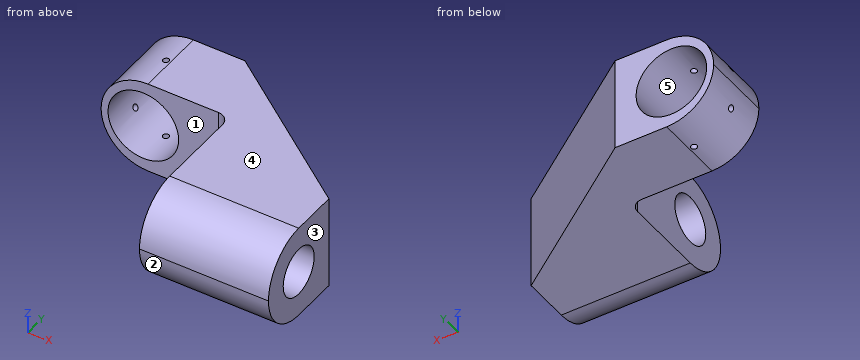
```python
from build123d import *

# Parameters (mm, degrees)
BOSS_EXTRUDE1_DEPTH     = 40
FILLET1_R               = 5
CUT_EXTRUDE1_REACH      = 114.805
SKETCH2_R               = 10.25
CUT_EXTRUDE2_REACH      = 133.529
SKETCH3_R               = 15.05
FILLET3_R               = 20
CUT_EXTRUDE5_DEPTH      = 37
CUT_EXTRUDE5_DEPTH_BACK = 7
SKETCH7_R               = 1.325
CUT_EXTRUDE7_DEPTH      = 7
CUT_EXTRUDE7_DEPTH_BACK = 7
SKETCH8_R               = 1.325
CUT_EXTRUDE8_DEPTH      = 7
CUT_EXTRUDE8_DEPTH_BACK = 7
SKETCH9_R               = 1.325
FILLET4_START           = -30
FILLET4_DEPTH           = 30


with BuildPart() as part:
    # Sketch1 → Boss-Extrude1 (new body)
    with BuildSketch(Plane.XY):
        Polygon((0, 0), (42, 0), (110, -50), (110, -90), (55, -90), (55, -30), (0, -30), align=None)
    extrude(amount=BOSS_EXTRUDE1_DEPTH)

    # Fillet1
    fillet1_edges = [part.edges().sort_by_distance(p)[0] for p in [
        (55, -30, 20),
    ]]
    fillet(fillet1_edges, radius=FILLET1_R)

    # Sketch2 → Cut-Extrude1 (cut, up to next)
    with BuildSketch(Plane.ZY.offset(-55), mode=Mode.PRIVATE) as cut_extrude1_sk1:
        with Locations((20, -70)):
            Circle(SKETCH2_R)
    cut_extrude1_tool1 = extrude(cut_extrude1_sk1.sketch, amount=-CUT_EXTRUDE1_REACH, mode=Mode.PRIVATE) & part.part
    add(cut_extrude1_tool1.solids().sort_by_distance((55, -70, 20))[0], mode=Mode.SUBTRACT)

    # Sketch3 → Cut-Extrude2 (cut, up to next)
    with BuildSketch(Plane.XZ.offset(30), mode=Mode.PRIVATE) as cut_extrude2_sk1:
        with Locations((18, 20)):
            Circle(SKETCH3_R)
    cut_extrude2_tool1 = extrude(cut_extrude2_sk1.sketch, amount=-CUT_EXTRUDE2_REACH, mode=Mode.PRIVATE) & part.part
    add(cut_extrude2_tool1.solids().sort_by_distance((18, -30, 20))[0], mode=Mode.SUBTRACT)

    # Fillet3
    fillet3_edges = [part.edges().sort_by_distance(p)[0] for p in [
        (82.5, -90, 0),
        (82.5, -90, 40),
    ]]
    fillet(fillet3_edges, radius=FILLET3_R - 0.0001)  # a hair under: the kernel refuses the full size

    # Sketch7 → Cut-Extrude5 (cut, two sides: drawn at the far end of the back side and taken through both)
    with BuildSketch(Plane.XY.offset(4.95).offset(-CUT_EXTRUDE5_DEPTH_BACK)):
        with Locations(Location((18, -15, 0), (0, 0, 180))):
            Circle(SKETCH7_R)
    extrude(amount=CUT_EXTRUDE5_DEPTH + CUT_EXTRUDE5_DEPTH_BACK, mode=Mode.SUBTRACT)

    # Sketch8 → Cut-Extrude7 (cut, two sides: drawn at the far end of the back side and taken through both)
    with BuildSketch(Plane(origin=(9.126571711, 0, 5.269228634), x_dir=(0.4999999999999973, 0, -0.8660254037844402), z_dir=(0.8660254037844403, 0, 0.4999999999999973)).offset(-CUT_EXTRUDE7_DEPTH_BACK)):
        with Locations(Location((-8.320508076, -15, 0), (0, 0, 180))):
            Circle(SKETCH8_R)
    extrude(amount=CUT_EXTRUDE7_DEPTH + CUT_EXTRUDE7_DEPTH_BACK, mode=Mode.SUBTRACT)

    # Sketch9 → Cut-Extrude8 (cut, two sides: drawn at the far end of the back side and taken through both)
    with BuildSketch(Plane(origin=(4.966317673, 0, 27.525), x_dir=(-0.49999999999999806, 0, -0.8660254037844399), z_dir=(0.8660254037844399, 0, -0.49999999999999806)).offset(-CUT_EXTRUDE8_DEPTH_BACK)):
        with Locations(Location((0, -15, 0), (0, 0, 180))):
            Circle(SKETCH9_R)
    extrude(amount=CUT_EXTRUDE8_DEPTH + CUT_EXTRUDE8_DEPTH_BACK, mode=Mode.SUBTRACT)

    # Fillet4: read off the stored shape, not the designer's step
    # Fillet4 outline → Fillet4 (cut)
    with BuildSketch(Plane(origin=(0, 0, 0), x_dir=(1, 0, 0), z_dir=(0, 1, 0)).offset(FILLET4_START)):
        with BuildLine():
            ThreePointArc((20, -40), (5.857864376, -34.142135624), (0, -20))
            Line((0, -20), (0, -40))
            Line((0, -40), (20, -40))
        make_face()
        with BuildLine():
            ThreePointArc((0, -20), (5.857864376, -5.857864376), (20, 0))
            Line((20, 0), (0, 0))
            Line((0, 0), (0, -20))
        make_face()
    extrude(amount=FILLET4_DEPTH, mode=Mode.SUBTRACT)


solid = part.part
```
Design review of the part built by this model. Coordinates are the model's own, in mm. Face numbers are marked on the shaded views. A direction names the side the tool comes from. Coordinates: 2 decimals unless noted, no trailing zeros. Loops run counter-clockwise (first coordinate to the right, second up) from the corner with the lowest first, then second, coordinate; pieces in that order, holes last. Notation, with made-up numbers: (74, 86.25) -> (127, 86.25) arc R22 ccw to (127, 124.25) -> close; hole circle Ø7 at (16, 61). An arc over 180 degrees is marked (long way). Answer as a JSON object with one key per item and string values.
Q1. Take a section at C-C on x = 18. Give the boundary of the cut face in (y, z) (3 decimals).
Answer block:
{"outline": "(-30, 0.1) -> (-16.325, 0.1) -> (-16.325, 4.95) -> (-30, 4.95) -> close; (-30, 35.05) -> (-16.325, 35.05) -> (-16.325, 39.9) -> (-30, 39.9) -> close; (-13.675, 0.1) -> (0, 0.1) -> (0, 4.95) -> (-13.675, 4.95) -> close; (-13.675, 35.05) -> (0, 35.05) -> (0, 39.9) -> (-13.675, 39.9) -> close"}
Q2. To check wall thickness, follow L1, parallel to Y at x = 18, z = 2.4 (3 decimals); L2, parallel to Z at x = 29, y = -16.5; L3, parallel to Y at x = 40.5, z = 2. State the ranges of each line that lie inside material, in increasing order.
Answer block:
{"L1": "y = -30 to -16.325, -13.675 to 0", "L2": "z = 0 to 9.73, 30.27 to 40", "L3": "y = -30 to 0"}
Q3. Tool access review of the marked faces 1 and 2: name each direction out of +Z, -Z, +X, -X, +Y, -Y from which nothing blocks a thin tool from reaching the whole face with its end or side.
Answer block:
{"face 1": "+Z, -Z, -X, -Y", "face 2": "-Z, +X, -X, -Y"}
Q4. Clearance check with flat-ended pins moving along their axes: pin 1 Ø1.5 at (x, z) = (63, 16.5) entering from +Y; pin 2 Ø10 at (x, z) = (59, 21.5) entering from +Y; pin 3 Ø1.5 at (x, z) = (61, 33.5) entering from +Y. State where each tip first meets the part, or that it passes through.
Answer block:
{"pin 1": "stops at y = -14.89", "pin 2": "stops at y = -8.82", "pin 3": "stops at y = -13.42"}
Q5. Take a section at D-D on z = 24. Give the boundary of the cut face in (x, y).
Answer block:
{"outline": "(0.4, -30) -> (3.49, -30) -> (3.49, 0) -> (0.4, 0) -> close; (32.51, -30) -> (50, -30) arc R5 cw to (55, -35) -> (55, -60.56) -> (110, -60.56) -> (110, -50) -> (42, 0) -> (32.51, 0) -> close; (55, -89.6) -> (110, -89.6) -> (110, -79.44) -> (55, -79.44) -> close"}
Q6. The part is to be moulded in two halves that separate along Z. For the marked faces 3, 4 and 5, say which applies: +Z half, -Z half, draft (parallel to the pull), parting line (faces both ways), or undercut.
Answer block:
{"face 3": "draft", "face 4": "+Z half", "face 5": "undercut"}
Q7. Take a section at A-A on y = -18. Give the boundary of the cut face in (x, z), plus the area to 3 significant figures.
Answer block:
{"outline": "(20, 0) -> (66.48, 0) -> (66.48, 40) -> (20, 40) arc R20 ccw to start; hole circle Ø30.1 at (18, 20)", "area": "1,780 mm^2"}
